The listing builds one solid part. Answer for the finished solid, in the listing's coordinates (mm). A direction names the side the tool comes from. Coordinates: 2 decimals unless noted, no trailing zeros. Order: outer loops, then holes, each group sorted by start corner. A loop starts at its lowest first (then second) coordinate and runs counter-clockwise, first axis right, second up. Notation, with made-up numbers: (4.5, 57.5) -> (59.5, 57.5) arc R10 ccw to (59.5, 70.5) -> close; hole circle Ø8 at (-15.75, 68.5). An arc over 180 degrees is marked (long way). Return JSON: item names as keys, results as strings.
from build123d import *

# Parameters (mm, degrees)
PAD_DEPTH    = 2
POCKET_DEPTH = 0.5
CHAMFER_SIZE = 0.25


with BuildPart() as part:
    # Sketch → Pad (new body)
    with BuildSketch(Plane.XY):
        Polygon((-5, -8.660254), (5, -8.660254), (10, 0), (5, 8.660254), (-5, 8.660254), (-10, 0), align=None)
    extrude(amount=PAD_DEPTH)

    # Sketch001 → Pocket (cut)
    with BuildSketch(Plane.XY.offset(2)):
        Polygon((4.42265, -7.660254), (8.845299, 0), (4.42265, 7.660254), (-4.42265, 7.660254), (-8.845299, 0), (-4.42265, -7.660254), align=None)
    extrude(amount=-POCKET_DEPTH, mode=Mode.SUBTRACT)

    # Chamfer
    chamfer_edges = [part.edges().sort_by_distance(p)[0] for p in [
        (0, -8.660254, 2),
        (-7.5, -4.330127, 2),
        (7.5, -4.330127, 2),
        (-7.5, 4.330127, 2),
        (7.5, 4.330127, 2),
        (0, 8.660254, 2),
        (0, -7.660254, 2),
        (-6.633975, -3.830127, 2),
        (-6.633975, 3.830127, 2),
        (0, 7.660254, 2),
        (6.633975, 3.830127, 2),
        (6.633975, -3.830127, 2),
    ]]
    chamfer(chamfer_edges, length=CHAMFER_SIZE)


solid = part.part
1. The part is cut by section B-B on z = 1.1. Give the vertices of the cut face in (x, y).
Answer block:
{"outline": "(-10, 0) -> (-5, -8.66) -> (5, -8.66) -> (10, 0) -> (5, 8.66) -> (-5, 8.66) -> close"}
2. The part is cut by section A-A on x = -4. Give the vertices of the cut face in (y, z), and give its area (3 significant figures).
Answer block:
{"outline": "(-8.66, 0) -> (8.66, 0) -> (8.66, 1.75) -> (8.41, 2) -> (7.91, 2) -> (7.66, 1.75) -> (7.66, 1.5) -> (-7.66, 1.5) -> (-7.66, 1.75) -> (-7.91, 2) -> (-8.41, 2) -> (-8.66, 1.75) -> close", "area": "26.9 mm2"}
3. For faces 4 (the face through (-7.465, 4.391, 0.863)), 5 (the face through (-6.709, 3.947, 1.873)), determine the directions among +Z, -Z, +X, -X, +Y, -Y from which every point of the face is accessible in a straight line to the end or side of a thin tool.
Answer block:
{"face 4": "+Z, -Z, -X, +Y", "face 5": "+Z"}
4. Consider line 1 (Z direction, x = -4.75, y = 4.5); line 2 (Y direction, x = -4, z = 1.9); line 3 (X direction, y = 4.5, z = 1.9). Determine where each line is inside the solid, lowest interval first. Write a range as from..to.
Answer block:
{"line 1": "z = 0..1.5", "line 2": "y = -8.51..-7.81, 7.81..8.51", "line 3": "x = -7.23..-6.42, 6.42..7.23"}
5. The part is cut by section C-C on y = -2. Give the vertices of the cut face in (x, z).
Answer block:
{"outline": "(-8.85, 0) -> (8.85, 0) -> (8.85, 1.75) -> (8.56, 2) -> (7.98, 2) -> (7.69, 1.75) -> (7.69, 1.5) -> (-7.69, 1.5) -> (-7.69, 1.75) -> (-7.98, 2) -> (-8.56, 2) -> (-8.85, 1.75) -> close"}
6. Determine the mould class of faces 1 (the face through (7.43, 4.21, 1.87)), 2 (the face through (-7.535, -4.27, 0.863)), 3 (the face through (6.709, -3.947, 1.873)) for opening direction Y: pulls with the +Y half, pulls with the -Y half, needs draft (parallel to the pull), parting line crosses it, or undercut.
Answer block:
{"face 1": "pulls with the +Y half", "face 2": "pulls with the -Y half", "face 3": "undercut"}
7. This flat-tipped pin is pushed along its axis until it touches: pin 1 Ø7.5 at (x, y) = (2.5, -2.5) entering from +Z. Where does it stop, or does it pass through?
Answer block:
{"pin 1": "stops at z = 1.5"}
